Here's how the part is built. I have some questions about the finished solid (model axes, mm). Round coordinates to 2 decimals unless told otherwise and drop trailing zeros. Order: outer loops, then holes, each group sorted by start corner. A loop starts at its lowest first (then second) coordinate and runs counter-clockwise, first axis right, second up. Notation, with made-up numbers: (6, -20.5) - (13, -20.5) arc R25 cw to (13, -5.5) - close; hole circle Ø4 at (47, -17). An arc over 180 degrees is marked (long way). Answer as a JSON object with one key per item and string values.
```python
from build123d import *

# Parameters (mm, degrees)
F0_W     = 150
F0_H     = 66
F1_DEPTH = 39.7
F2_W     = 150
F2_H     = 7
F3_DEPTH = 30
F2_H_2   = 8
F4_DEPTH = 30
F5_DEPTH = 30
F6_DEPTH = 30
F7_DEPTH = 30
F8_DEPTH = 30


with BuildPart() as f1:
    # F0 (on Front) → F1 (new body)
    with BuildSketch(Plane.XZ):
        with Locations((-68.706734, 1.151069)):
            Rectangle(F0_W, F0_H)
    extrude(amount=F1_DEPTH)

    # F2 (on face) → F3 (cut)
    with BuildSketch(Plane.XZ.offset(39.7)):
        with Locations((-68.706734, 26.651069)):
            Rectangle(F2_W, F2_H)
    extrude(amount=-F3_DEPTH, mode=Mode.SUBTRACT)

    # F2 (on face) → F4 (cut)
    with BuildSketch(Plane.XZ.offset(39.7)):
        with Locations((-68.706734, 16.551069)):
            Rectangle(F2_W, F2_H_2)
    extrude(amount=-F4_DEPTH, mode=Mode.SUBTRACT)

    # F2 (on face) → F5 (cut)
    with BuildSketch(Plane.XZ.offset(39.7)):
        with Locations((-68.706734, 5.951069)):
            Rectangle(F2_W, F2_H_2)
    extrude(amount=-F5_DEPTH, mode=Mode.SUBTRACT)

    # F2 (on face) → F6 (cut)
    with BuildSketch(Plane.XZ.offset(39.7)):
        with Locations((-68.706734, -4.648931)):
            Rectangle(F2_W, F2_H_2)
    extrude(amount=-F6_DEPTH, mode=Mode.SUBTRACT)

    # F2 (on face) → F7 (cut)
    with BuildSketch(Plane.XZ.offset(39.7)):
        with Locations((-68.706734, -15.248931)):
            Rectangle(F2_W, F2_H_2)
    extrude(amount=-F7_DEPTH, mode=Mode.SUBTRACT)

    # F2 (on face) → F8 (cut)
    with BuildSketch(Plane.XZ.offset(39.7)):
        with Locations((-68.706734, -25.848931)):
            Rectangle(F2_W, F2_H_2)
    extrude(amount=-F8_DEPTH, mode=Mode.SUBTRACT)


solid = f1.part
```
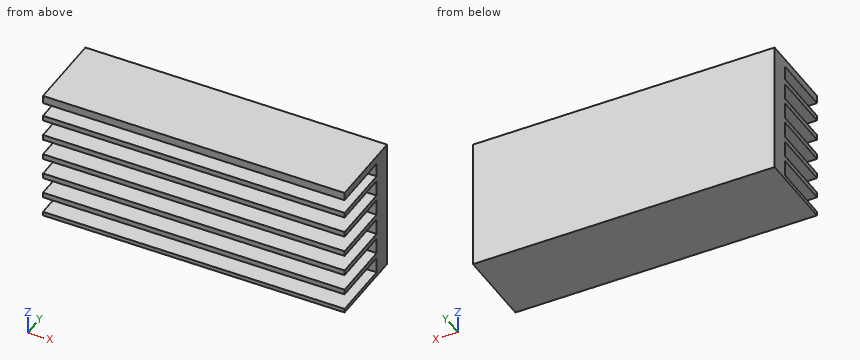
1. Imagine slicing it at A-A (y = -24). List the corners of the cut face in (x, z) for me, plus the area to 3 significant figures.
Responses:
{"outline": "(-143.71, -31.85) - (6.29, -31.85) - (6.29, -29.85) - (-143.71, -29.85) - close; (-143.71, -21.85) - (6.29, -21.85) - (6.29, -19.25) - (-143.71, -19.25) - close; (-143.71, -11.25) - (6.29, -11.25) - (6.29, -8.65) - (-143.71, -8.65) - close; (-143.71, -0.65) - (6.29, -0.65) - (6.29, 1.95) - (-143.71, 1.95) - close; (-143.71, 9.95) - (6.29, 9.95) - (6.29, 12.55) - (-143.71, 12.55) - close; (-143.71, 20.55) - (6.29, 20.55) - (6.29, 23.15) - (-143.71, 23.15) - close; (-143.71, 30.15) - (6.29, 30.15) - (6.29, 34.15) - (-143.71, 34.15) - close", "area": "2,850 mm2"}
2. Imagine slicing it at C-C (z = 26.5). List the corners of the cut face in (x, y) for me.
Responses:
{"outline": "(-143.71, -9.7) - (6.29, -9.7) - (6.29, 0) - (-143.71, 0) - close"}
3. Imagine slicing it at B-B (x = -58). List the corners of the cut face in (y, z) for me, plus the area to 3 significant figures.
Responses:
{"outline": "(-39.7, -31.85) - (0, -31.85) - (0, 34.15) - (-39.7, 34.15) - (-39.7, 30.15) - (-9.7, 30.15) - (-9.7, 23.15) - (-39.7, 23.15) - (-39.7, 20.55) - (-9.7, 20.55) - (-9.7, 12.55) - (-39.7, 12.55) - (-39.7, 9.95) - (-9.7, 9.95) - (-9.7, 1.95) - (-39.7, 1.95) - (-39.7, -0.65) - (-9.7, -0.65) - (-9.7, -8.65) - (-39.7, -8.65) - (-39.7, -11.25) - (-9.7, -11.25) - (-9.7, -19.25) - (-39.7, -19.25) - (-39.7, -21.85) - (-9.7, -21.85) - (-9.7, -29.85) - (-39.7, -29.85) - close", "area": "1,210 mm2"}
4. For P1, Ø12, axis at x = -43.5, z = -5, coming from the -Y side; P2, Ø3.5, axis at x = -51, z = 28, coming from the -Y side; P3, Ø5, axis at y = -24, z = -4.5, coming from the -X side, each with a flat end and sliding along its axis, tell me the tip position at first contact or that it passes through.
Responses:
{"P1": "y = -39.7", "P2": "y = -9.7", "P3": "through"}
5. If I drill on L1, parallel to Y at x = -129, z = 5.5, over which ranges is the centre line in solid material (lowest first)? Write a range as [from, to].
Responses:
{"L1": "[-9.7, 0]"}
